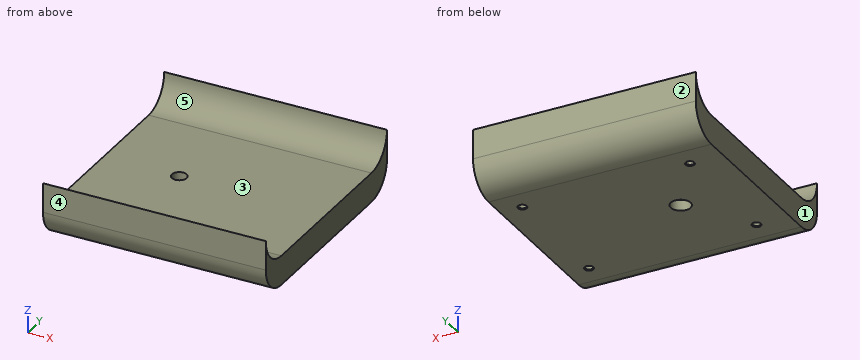
Autodesk Inventor part; units mm, degrees
ref_plane "YZ Plane" through (0, 0, 0) normal (1, 0, 0) x (0, 1, 0)
ref_plane "XZ Plane" through (0, 0, 0) normal (0, 1, 0) x (-1, 0, 0)
ref_plane "XY Plane" through (0, 0, 0) normal (0, 0, 1) x (1, 0, 0)
ref_plane "作業平面1" through (-27.3255, 41.0319, 38.0074) normal (1, 0, 0) x (0, 1, 0)
sketch "スケッチ2" plane through (-27.3255, 41.0319, 38.0074) normal (1, 0, 0) x (0, 1, 0)
  arc A0 (-51.6, -13.3) -> (-38.35, -26.55) centre (-38.35, -13.3) ccw
  line L0 (-51.6, 0) -> (-51.6, -13.3)
  arc A1 (-51.6, 0) -> (-38.35, -13.25) centre (-38.35, 0) ccw
  line L1 (38.35, -13.25) -> (-38.35, -13.25)
  arc A2 (38.35, -13.25) -> (51.6, 0) centre (38.35, 0) ccw
  line L2 (51.6, -13.3) -> (51.6, 0)
  arc A3 (38.35, -26.55) -> (51.6, -13.3) centre (38.35, -13.3) ccw
  line L3 (-38.35, -26.55) -> (38.35, -26.55)
  point P0 (-41.0319, -38.0074)
extrude "押し出し1" add sketch "スケッチ2" along normal blind 100.9
sketch "スケッチ3" plane through (-27.3255, 2.6819, 11.4574) normal (0, 0, -1) x (-1, 0, 0)
  line L0 (0, 76.7) -> (-100.9, 76.7)
  line L1 (-100.9, 0) -> (-100.9, 76.7)
  line L2 (0, 0) -> (-100.9, 0)
  line L3 (0, 76.7) -> (0, 0)
  point P0 (-27.3255, -2.6819)
  point P1 (-90.9, 66.7)
  point P2 (-90.9, 10)
  point P3 (-15, 10)
  point P4 (-15, 66.7)
  dimension "d2" = 10
  dimension "d3" = 10
  dimension "d4" = 10
  dimension "d5" = 10
  dimension "d6" = 10
  dimension "d7" = 15
  dimension "d8" = 15
  dimension "d9" = 10
hole "穴2" at (63.5745, 69.3819, 11.4574) at (63.5745, 12.6819, 11.4574) at (-12.3255, 12.6819, 11.4574) at (-12.3255, 69.3819, 11.4574) direction (0, 0, 1) diameter 3.3 depth 10.979 tip angle 118 countersink diameter 4 countersink angle 90
sketch "スケッチ4" plane through (-27.3255, 2.6819, 11.4574) normal (0, 0, -1) x (-1, 0, 0)
  circle A0 centre (-34.275, 38.35) radius 4.175
  circle A1 centre (-34.275, 38.35) radius 3.35
  point P0 (-27.3255, -2.6819)
  dimension "d24" = 6.7
hole "穴3" at (6.9495, 41.0319, 11.4574) direction (0, 0, 1) diameter 6.7 depth 15 tip angle 118 counterbore diameter 9 counterbore depth 5
properties part number "AzureKinectCradle"
Read the model definition and answer for the solid it produces. Units are mm, in the model's axes. Face numbers are marked on the shaded views. A direction names the side the tool comes from. Round coordinates to 2 decimals unless told otherwise and drop trailing zeros. Write each loop counter-clockwise with the first axis right and the second up, starting at its lowest first coordinate (ties: lowest second). Pieces come first, ordered by that corner, then holes. Notation, with made-up numbers: (-16, 35) -> (19, 35) arc R27 cw to (19, 68) -> close; hole circle Ø11 at (-10, 30.5). An arc over 180 degrees is marked (long way). Answer in a Markdown table with one row per item. Add a question column.
1) Given P1, Ø2.5, axis at x = -12.33, y = 69.38, coming from the +Z side; P2, Ø2, axis at x = 7.5, z = 21.5, coming from the -Y side; P3, Ø2, axis at x = 63.57, y = 12.68, coming from the -Z side, each flat-ended and moving along its own axis, determine where each tip first touches the part or whether it passes through.
2) Find section B-B, the plane x = 5. Determine the outline of the cut face in (y, z).
3) Determine the mould class of the marked faces 1, 2 and 3 for opening direction Y: pulls with the +Y half, pulls with the -Y half, needs draft (parallel to the pull), parting line crosses it, or undercut.
4) Find section D-D, the plane y = 86.5. Determine the outline of the cut face in (x, z), and give its area (3 significant figures).
5) Consider line 1 (Z direction, x = -11, y = 8.5); line 2 (Y direction, x = -6, z = 33.5); line 3 (Y direction, x = 9, z = 23.25). Determine where each line is inside the solid, lowest interval first.
6) Find section A-A, the plane z = 28.25. Determine the outline of the cut face in (x, y), and give its area (3 significant figures).
7) Which of the six approach directions +Z, -Z, +X, -X, +Y, -Y give full straight-line access (tool end or side, diameter ignored) to the marked faces 4 and 5?
8) Find section C-C, the plane z = 14. Determine the outline of the cut face in (x, y).
Findings below:
| question | item | result |
|---|---|---|
| 1 | P1 | z = 24.76 |
| 1 | P2 | y = -10.38 |
| 1 | P3 | z = 22.82 |
| 2 | outline | (-10.57, 24.71) arc R13.25 ccw to (2.68, 11.46) -> (36.98, 11.46) -> (36.98, 16.46) -> (38.31, 16.46) -> (38.31, 24.76) -> (2.68, 24.76) arc R13.25 cw to (-10.57, 38.01) -> close; (43.76, 16.46) -> (45.09, 16.46) -> (45.09, 11.46) -> (79.38, 11.46) arc R13.25 ccw to (92.63, 24.71) -> (92.63, 38.01) arc R13.25 cw to (79.38, 24.76) -> (43.76, 24.76) -> close |
| 3 | face 1 | needs draft |
| 3 | face 2 | pulls with the +Y half |
| 3 | face 3 | undercut |
| 4 | outline | (-27.33, 13.53) -> (73.57, 13.53) -> (73.57, 26.83) -> (-27.33, 26.83) -> close |
| 4 | area | 1,340 mm² |
| 5 | line 1 | 11.46 to 24.76 |
| 5 | line 2 | -10.57 to -9.78, 91.84 to 92.63 |
| 5 | line 3 | -10.49 to 38.38, 43.68 to 92.55 |
| 6 | outline | (-27.33, -10.57) -> (73.57, -10.57) -> (73.57, -6.28) -> (-27.33, -6.28) -> close; (-27.33, 88.35) -> (73.57, 88.35) -> (73.57, 92.63) -> (-27.33, 92.63) -> close |
| 6 | area | 865 mm² |
| 7 | face 4 | +Z, -Z, +X, -X, -Y |
| 7 | face 5 | +Z, +X, -X |
| 8 | outline | (-27.33, -5.12) -> (73.57, -5.12) -> (73.57, 87.19) -> (-27.33, 87.19) -> close; hole circle Ø3.3 at (-12.33, 12.68); hole circle Ø3.3 at (-12.33, 69.38); hole circle Ø9 at (6.95, 41.03); hole circle Ø3.3 at (63.57, 12.68); hole circle Ø3.3 at (63.57, 69.38) |
